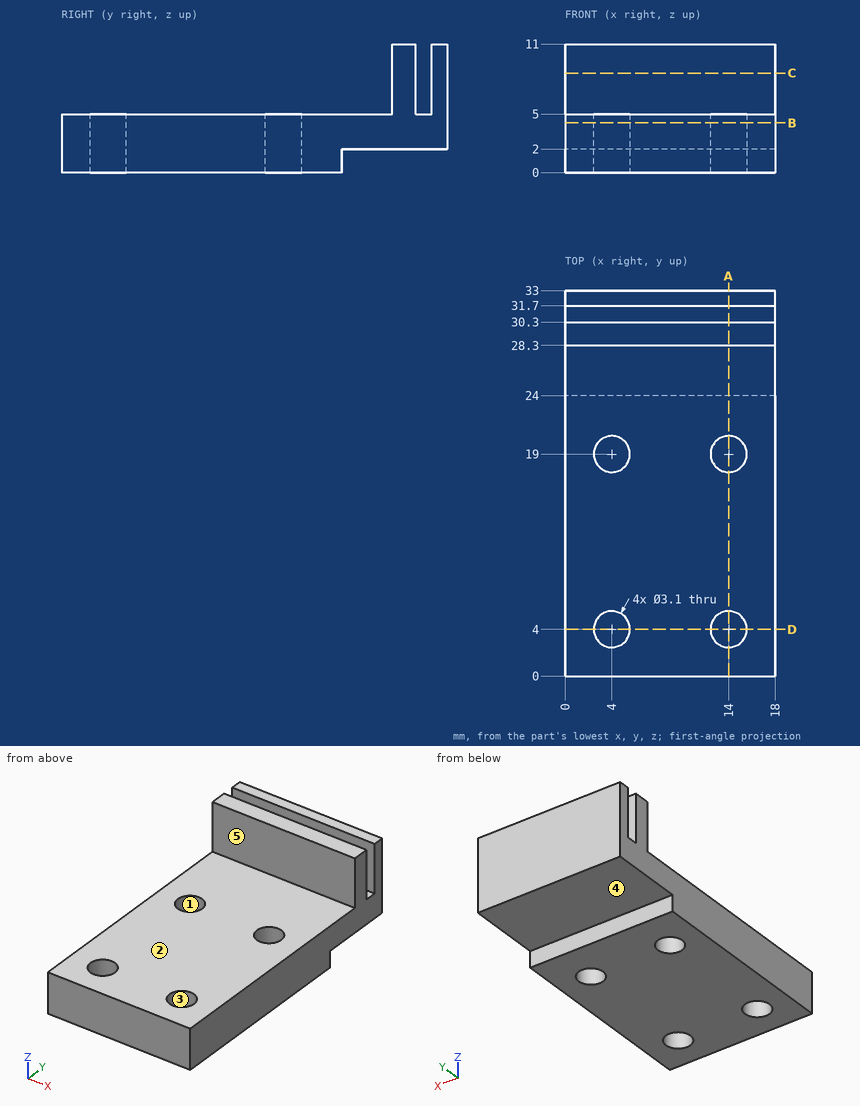
Could you check a few things on this drawing? It's one solid part, dimensions in mm from its lowest x, y, z. A direction names the side the tool comes from. Coordinates: 2 decimals unless noted, no trailing zeros. Write each loop counter-clockwise with the first axis right and the second up, starting at its lowest first coordinate (ties: lowest second). Pieces come first, ordered by that corner, then holes.
Q1. Please list where these lines run through material, in increasing order: L1, parallel to Y at x = 14, z = 1.35; L2, parallel to Y at x = 14, z = 3.85; L3, parallel to Y at x = 1, z = 9.25.
Results found:
L1: y = 0 to 2.45, 5.55 to 17.45, 20.55 to 24
L2: y = 0 to 2.45, 5.55 to 17.45, 20.55 to 33
L3: y = 28.3 to 30.3, 31.7 to 33
Q2. Which directions (+Z, -Z, +X, -X, +Y, -Y) give clear straight access to the entire face, cutting with the end or side of a thin tool? Please do the marked faces 1 and 2.
Results found:
face 1: +Z, -Z
face 2: +Z, +X, -X, -Y
Q3. Imagine slicing it at D-D, the plane y = 4. List the corners of the cut face in (x, z) for me, plus the area to 3 significant figures.
Results found:
outline: (0, 0) - (2.45, 0) - (2.45, 5) - (0, 5) - close; (5.55, 0) - (12.45, 0) - (12.45, 5) - (5.55, 5) - close; (15.55, 0) - (18, 0) - (18, 5) - (15.55, 5) - close
area: 59.0 mm2
Q4. If we mould it in two halves opening along Y, with no side actions, what happens to the marked faces 3, 4 and 5? For each: +Y half, -Y half, draft (parallel to the pull), parting line (faces both ways), or undercut.
Results found:
face 3: undercut
face 4: draft
face 5: -Y half
Q5. Imagine slicing it at A-A, the plane x = 14. List the corners of the cut face in (y, z) for me, plus the area to 3 significant figures.
Results found:
outline: (0, 0) - (2.45, 0) - (2.45, 5) - (0, 5) - close; (5.55, 0) - (17.45, 0) - (17.45, 5) - (5.55, 5) - close; (20.55, 0) - (24, 0) - (24, 2) - (33, 2) - (33, 11) - (31.7, 11) - (31.7, 5) - (30.3, 5) - (30.3, 11) - (28.3, 11) - (28.3, 5) - (20.55, 5) - close
area: 136 mm2
Q6. Imagine slicing it at C-C, the plane z = 8.5. List the corners of the cut face in (x, y) for me, plus the area to 3 significant figures.
Results found:
outline: (0, 28.3) - (18, 28.3) - (18, 30.3) - (0, 30.3) - close; (0, 31.7) - (18, 31.7) - (18, 33) - (0, 33) - close
area: 59.4 mm2
Q7. For P1, Ø0.7, axis at x = 12, y = 31, coming from the +Z side; P2, Ø3, axis at y = 27, z = 7, coming from the -X side; P3, Ø4.5, axis at x = 5.5, y = 29, coming from the -Z side; P4, Ø1.8, axis at x = 11, z = 7, coming from the -Y side, each with a flat end and sliding along its axis, tell me the tip position at first contact or that it passes through.
Results found:
P1: stops at z = 5
P2: stops at x = 0
P3: stops at z = 2
P4: stops at y = 28.3
Q8. Imagine slicing it at B-B, the plane z = 4.25. List the corners of the cut face in (x, y) for me, plus the area to 3 significant figures.
Results found:
outline: (0, 0) - (18, 0) - (18, 33) - (0, 33) - close; hole circle Ø3.1 at (4, 4); hole circle Ø3.1 at (4, 19); hole circle Ø3.1 at (14, 4); hole circle Ø3.1 at (14, 19)
area: 564 mm2
